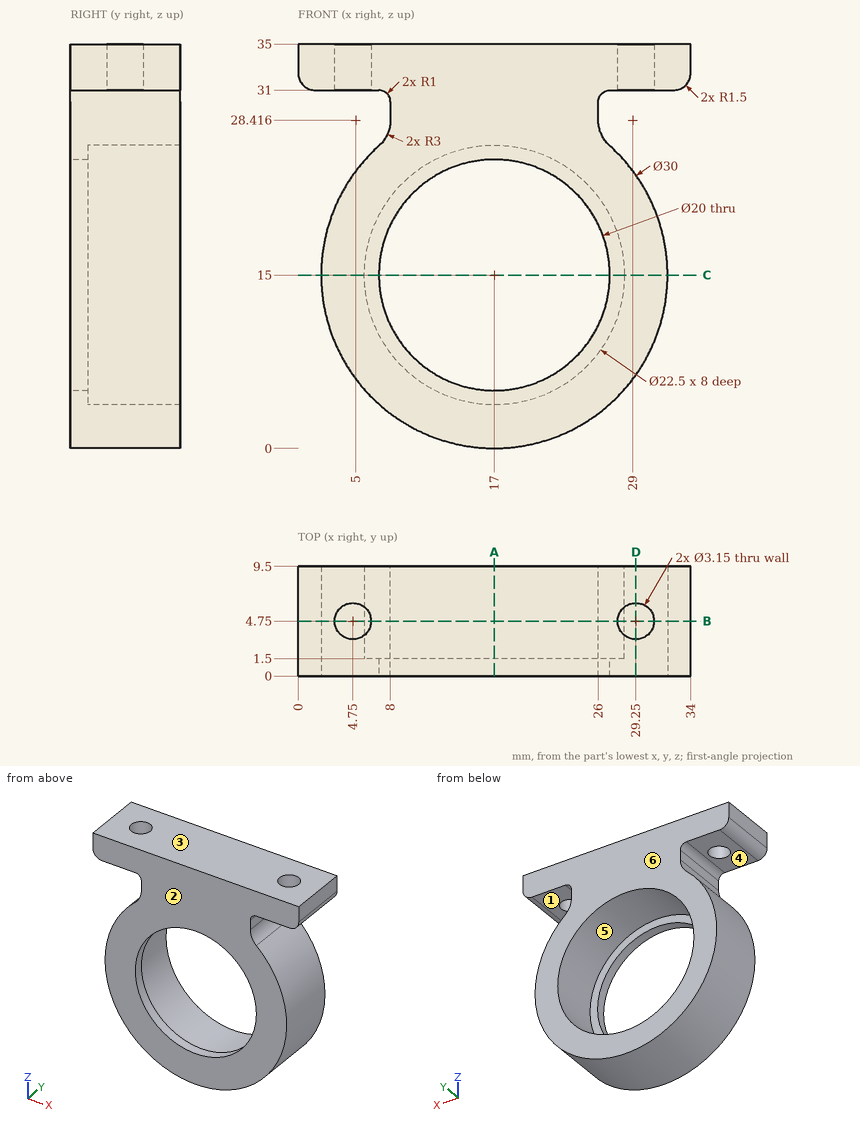
Answer from the drawing. Dimensions are ordinates in mm from the lowest x, y and z of the part. A direction names the side the tool comes from. Round coordinates to 2 decimals unless told otherwise and drop trailing zeros. Write each loop counter-clockwise with the first axis right and the second up, starting at its lowest first coordinate (ties: lowest second). Pieces come first, ordered by that corner, then holes. Notation, with made-up numbers: (47.25, 15.5) -> (99.25, 15.5) arc R18 cw to (99.25, 29.5) -> close; hole circle Ø2 at (-36, -5). An arc over 180 degrees is marked (long way). Write each question's results on one line, items separated by ' | '.
1) The part is cut by section A-A (x = 17). Write down the section's boundary in (y, z).
Findings:
outline: (0, 0) -> (9.5, 0) -> (9.5, 3.75) -> (1.5, 3.75) -> (1.5, 5) -> (0, 5) -> close; (0, 25) -> (1.5, 25) -> (1.5, 26.25) -> (9.5, 26.25) -> (9.5, 35) -> (0, 35) -> close
2) For a pull along Z with two mould halves and no side action, classify the marked faces 1, 2, 3 and 4 as +Z half, -Z half, draft (parallel to the pull), parting line (faces both ways), or undercut.
Findings:
face 1: undercut | face 2: draft | face 3: +Z half | face 4: undercut
3) Flat-ended cylindrical pins translate along their axes: pin 1 (5 mm diameter, centred on x = 29.25, y = 4.75, fed in from -Z); pin 2 (4.5 mm diameter, centred on x = 30, y = 3.5, fed in from -Z); pin 3 (1.7 mm diameter, centred on y = 6, z = 29, fed in from -X). Find the tip coordinate at first contact, or state that the pin passes through.
Findings:
pin 1: stops at z = 3.6 | pin 2: stops at z = 4.54 | pin 3: stops at x = 7.99
4) The part is cut by section B-B (y = 4.75). State how many separate pieces and enclosed holes the cut face has, and give its area (3 significant figures).
Findings:
separate pieces: 3 | enclosed holes: 1 | area: 455 mm²
5) The part is cut by section C-C (z = 15). Write down the section's boundary in (x, y).
Findings:
outline: (2, 0) -> (7, 0) -> (7, 1.5) -> (5.75, 1.5) -> (5.75, 9.5) -> (2, 9.5) -> close; (27, 0) -> (32, 0) -> (32, 9.5) -> (28.25, 9.5) -> (28.25, 1.5) -> (27, 1.5) -> close
6) Which of the six approach directions +Z, -Z, +X, -X, +Y, -Y give full straight-line access (tool end or side, diameter ignored) to the marked faces 5 and 6?
Findings:
face 5: +Y | face 6: +Z, -Z, +X, -X, +Y
7) Consider line 1 along Z through (x, y) = (17, 1.15); line 2 along Y through (x, z) = (4.75, 33.4) (1 decimal); line 3 along X through (y, z) = (3.5, 15). Determine where each line is inside the solid, lowest interval first. Write a range as [from, to].
Findings:
line 1: z = [0, 5], [25, 35] | line 2: y = [0, 3.2], [6.3, 9.5] | line 3: x = [2, 5.75], [28.25, 32]
8) The part is cut by section D-D (x = 29.25). Write down the section's boundary in (y, z) (1 decimal), and give its area (3 significant figures).
Findings:
outline: (0, 6.3) -> (9.5, 6.3) -> (9.5, 23.7) -> (0, 23.7) -> close; (0, 31) -> (3.2, 31) -> (3.2, 35) -> (0, 35) -> close; (6.3, 31) -> (9.5, 31) -> (9.5, 35) -> (6.3, 35) -> close | area: 190 mm²
